from build123d import *

# Parameters (mm, degrees)
SKETCH1_R           = 68
SKETCH1_R_2         = 63
BOSS_EXTRUDE1_DEPTH = 200
SCALE1_SCALE        = 0.560294118
CUT_EXTRUDE1_START  = -10
SKETCH2_R           = 38.1
SKETCH2_R_2         = 36.048529411
CUT_EXTRUDE1_DEPTH  = 10
BOSS_EXTRUDE2_START = 237.94
SKETCH3_R           = 38.1
SKETCH3_R_2         = 35.298529411
BOSS_EXTRUDE2_DEPTH = 237.94
SKETCH4_R           = 37.2
CUT_EXTRUDE2_DEPTH  = 349.998823528


with BuildPart() as part:
    # Sketch1 → Boss-Extrude1 (new body)
    with BuildSketch(Plane(origin=(0, 0, 0), x_dir=(1, 0, 0), z_dir=(0, 1, 0))):
        with Locations(Location((0, 0, 0), (0, 0, 270))):
            Circle(SKETCH1_R)
        with Locations(Location((0, 0, 0), (0, 0, 270))):
            Circle(SKETCH1_R_2, mode=Mode.SUBTRACT)
    extrude(amount=BOSS_EXTRUDE1_DEPTH)


with BuildPart() as part_1:
    # Scale1: scaled about (0, 100, 0)
    add(part.part.scale(SCALE1_SCALE).moved(Location((0, 43.970588236, 0))))

    # Sketch2 → Cut-Extrude1 (cut)
    with BuildSketch(Plane(origin=(0, 156.029411764, 0), x_dir=(1, 0, 0), z_dir=(0, 1, 0)).offset(CUT_EXTRUDE1_START)):
        with Locations(Location((0, 0, 0), (0, 0, 270))):
            Circle(SKETCH2_R)
        with Locations(Location((0, 0, 0), (0, 0, 270))):
            Circle(SKETCH2_R_2, mode=Mode.SUBTRACT)
    extrude(amount=CUT_EXTRUDE1_DEPTH, mode=Mode.SUBTRACT)

    # Sketch3 → Boss-Extrude2 (add)
    with BuildSketch(Plane.XZ.offset(-43.970588236).offset(BOSS_EXTRUDE2_START)):
        with Locations(Location((0, 0, 0), (0, 0, 270))):
            Circle(SKETCH3_R)
        with Locations(Location((0, 0, 0), (0, 0, 270))):
            Circle(SKETCH3_R_2, mode=Mode.SUBTRACT)
    extrude(amount=-BOSS_EXTRUDE2_DEPTH)

    # Sketch4 → Cut-Extrude2 (cut)
    with BuildSketch(Plane.XZ.offset(193.969411764)):
        with Locations(Location((0, 0, 0), (0, 0, 270))):
            Circle(SKETCH4_R)
    extrude(amount=-CUT_EXTRUDE2_DEPTH, mode=Mode.SUBTRACT)


solid = part_1.part
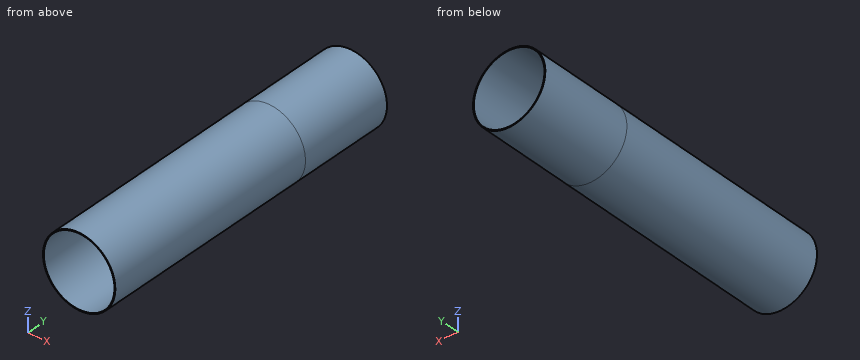
Input: part model. Units: mm. Frame: model coordinates. Round coordinates to 2 decimals unless told otherwise and drop trailing zeros. Loops run counter-clockwise (first coordinate to the right, second up) from the corner with the lowest first, then second, coordinate; pieces in that order, holes last. Notation, with made-up numbers: (66.5, 21.25) -> (90.5, 21.25) arc R23 cw to (90.5, 29.25) -> close; hole circle Ø1 at (48, -25.75). An arc over 180 degrees is marked (long way). Answer as a JSON object with one key per item and string values. Group by question number.
1) Section query A-A on z = 0. Output: boundary loops of the cut face in (x, y), plus the area to 3 significant figures.
2) Section query C-C on y = 38.5. Output: boundary loops of the cut face in (x, z), plus the area to 3 significant figures.
3) Ray query, L1, parallel to X at y = -54.5, z = 0; L2, parallel to Z at x = -8.5, y = -73; L3, parallel to Z at x = -5.5, y = -26. Return the intervals inside material, ascending.
4) Section query B-B on x = 0. Output: boundary loops of the cut face in (y, z), plus the area to 3 significant figures.
5) Pin query (flat end, axial travel): pin 1 (12 mm diameter, centred on y = 36.5, z = -1, fed in from -X); pin 2 (5 mm diameter, centred on x = -19.5, y = -112, fed in from -Z); pin 3 (2 mm diameter, centred on y = 76, z = 6.5, fed in from -X). Return the tip coordinate at first contact, or that it passes through.
Reply:
{
 "1": {"outline": "(-38.1, -193.97) -> (-37.2, -193.97) -> (-37.2, 146.03) -> (-38.1, 146.03) -> close; (37.2, -193.97) -> (38.1, -193.97) -> (38.1, 146.03) -> (37.2, 146.03) -> close", "area": "612 mm2"},
 "2": {"outline": "circle Ø76.2 at (0, 0); hole circle Ø74.4 at (0, 0)", "area": "213 mm2"},
 "3": {"L1": "x = -38.1 to -37.2, 37.2 to 38.1", "L2": "z = -37.14 to -36.22, 36.22 to 37.14", "L3": "z = -37.7 to -36.79, 36.79 to 37.7"},
 "4": {"outline": "(-193.97, -38.1) -> (146.03, -38.1) -> (146.03, -37.2) -> (-193.97, -37.2) -> close; (-193.97, 37.2) -> (146.03, 37.2) -> (146.03, 38.1) -> (-193.97, 38.1) -> close", "area": "612 mm2"},
 "5": {"pin 1": "stops at x = -38.1", "pin 2": "stops at z = -34.1", "pin 3": "stops at x = -37.7"}
}
